Autodesk Inventor part; units mm, degrees
ref_plane "YZ Plane" through (0, 0, 0) normal (1, 0, 0) x (0, 1, 0)
ref_plane "XZ Plane" through (0, 0, 0) normal (0, 1, 0) x (-1, 0, 0)
ref_plane "XY Plane" through (0, 0, 0) normal (0, 0, 1) x (1, 0, 0)
sketch "Sketch1" plane through (0, 0, 0) normal (0, 1, 0) x (-1, 0, 0)
  line L0 (0, 0) -> (-25.4, 0)
  line L1 (-25.4, 0) -> (-25.4, -3.175)
  line L2 (-25.4, -3.175) -> (0, -3.175)
  line L3 (0, -3.175) -> (0, 0)
  line L4 (-25.4, 0) -> (-22.225, 0)
  line L5 (-22.225, 0) -> (-22.225, -25.4)
  line L6 (-22.225, -25.4) -> (-25.4, -25.4)
  line L7 (-25.4, -25.4) -> (-25.4, 0)
  dimension "d0" = 25.4
  dimension "d1" = 3.175
  dimension "d2" = 25.4
  dimension "d3" = 3.175
extrude "Extrusion1" add sketch "Sketch1" along normal blind 152.4
sketch "Sketch2" plane through (22.225, 0, -25.4) normal (-1, 0, 0) x (0, 0, 1)
  line L0 (0, 0) -> (12.7, 0)
  line L1 (25.4, 0) -> (0, 0)
sketch "Sketch3" plane through (22.225, 0, -3.175) normal (0, 0, -1) x (-1, 0, 0)
  line L0 (0, 0) -> (22.225, 0)
  line L1 (22.225, 0) -> (11.1125, 0)
  line L2 (11.1125, 0) -> (11.1125, 38.1)
  line L3 (11.1125, 38.1) -> (11.1125, 114.3)
  circle A0 centre (11.1125, 38.1) radius 2.54
  circle A1 centre (11.1125, 114.3) radius 2.54
  dimension "d6" = 38.1
  dimension "d7" = 76.2
  dimension "d8" = 5.08
extrude "Extrusion2" cut sketch "Sketch3" against normal blind 25.4
properties part number "L Bracket 6in" material "Aluminum 6061"
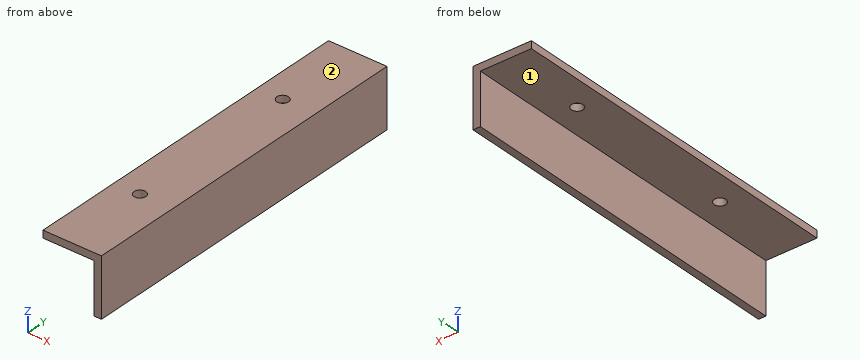
Can you work these out from the model? Positions are in its coordinate system, mm. Face numbers are marked on the shaded views. A direction names the side the tool comes from. Give positions to 0.01 mm unless a question says otherwise; leave off trailing zeros. Order: outer loops, then holes, each group sorted by start corner. A loop starts at its lowest first (then second) coordinate and runs counter-clockwise, first axis right, second up. Notation, with made-up numbers: (-19.5, 81) - (-15.5, 81) arc R22 ccw to (-15.5, 104) - close; hole circle Ø3 at (6, -26). An arc over 180 degrees is marked (long way). Use a Markdown table: item, result. Add a question column.
Q1. Please list where these lines run through material, in increasing order: line 1 along X through (y, z) = (114.3, -2.1); line 2 along Z through (x, y) = (9, 31) (3 decimals); line 3 along X through (y, z) = (14.5, -11.25) (3 decimals).
Q2. On a 3-axis mill with a long thin cutter (end or side, diameter ignored), from which of +Z, -Z, +X, -X, +Y, -Y can I reach the whole of each face in a straight line? I mean the marked faces 1 and 2. Say none if no direction works.
Q3. I'm going to push flat-ended pins straight in: pin 1 (4 mm diameter, centred on x = 11.11, y = 38.1, fed in from -Z); pin 2 (8 mm diameter, centred on x = 11.11, y = 114.3, fed in from -Z) (3 decimals); pin 3 (5 mm diameter, centred on y = 50, z = -20, fed in from -X) (3 decimals). Where does each tip first touch, or does it pass through?
Q4. If we section it at C-C on y = 82.5: Write out the boundary of the cut face in (x, z) (3 decimals), plus the area to 3 significant figures.
Q5. If we section it at D-D on z = -23.25: Write out the boundary of the cut face in (x, y) (3 decimals), plus the area to 3 significant figures.
Q6. If we section it at B-B on x = 10: Write out the boundary of the cut face in (y, z) (3 decimals), plus the area to 3 significant figures.
Q7. If we section it at A-A on y = 114.3: Write out the boundary of the cut face in (x, z) (1 decimal).
Answers follow:
| question | item | result |
|---|---|---|
| 1 | line 1 | x = 0 to 8.57, 13.65 to 25.4 |
| 1 | line 2 | z = -3.175 to 0 |
| 1 | line 3 | x = 22.225 to 25.4 |
| 2 | face 1 | -Z, -X, +Y, -Y |
| 2 | face 2 | +Z, +X, -X, +Y, -Y |
| 3 | pin 1 | passes through |
| 3 | pin 2 | stops at z = -3.175 |
| 3 | pin 3 | stops at x = 22.225 |
| 4 | outline | (0, -3.175) - (22.225, -3.175) - (22.225, -25.4) - (25.4, -25.4) - (25.4, 0) - (0, 0) - close |
| 4 | area | 151 mm^2 |
| 5 | outline | (22.225, 0) - (25.4, 0) - (25.4, 152.4) - (22.225, 152.4) - close |
| 5 | area | 484 mm^2 |
| 6 | outline | (0, -3.175) - (35.817, -3.175) - (35.817, 0) - (0, 0) - close; (40.383, -3.175) - (112.017, -3.175) - (112.017, 0) - (40.383, 0) - close; (116.583, -3.175) - (152.4, -3.175) - (152.4, 0) - (116.583, 0) - close |
| 6 | area | 455 mm^2 |
| 7 | outline | (0, -3.2) - (8.6, -3.2) - (8.6, 0) - (0, 0) - close; (13.7, -3.2) - (22.2, -3.2) - (22.2, -25.4) - (25.4, -25.4) - (25.4, 0) - (13.7, 0) - close |
